Geometry: final body of the model. Coordinates: model frame, mm. A direction names the side the tool comes from. Give positions to 0.01 mm unless a question says otherwise; leave off trailing zeros. Loops run counter-clockwise (first coordinate to the right, second up) from the corner with the lowest first, then second, coordinate; pieces in that order, holes last.
from build123d import *

# Parameters (mm, degrees)
BOSS_EXTRUDE1_DEPTH = 6
SKETCH2_R           = 5.75
BOSS_EXTRUDE2_DEPTH = 12
SKETCH4_R           = 2
CUT_EXTRUDE2_DEPTH  = 21.199009877
SKETCH5_R           = 1.5
CUT_EXTRUDE3_DEPTH  = 6


with BuildPart() as part:
    # Sketch1 → Boss-Extrude1 (new body)
    with BuildSketch(Plane(origin=(0, 0, 0), x_dir=(0, 1, 0), z_dir=(0, 0, 1))):
        Polygon((0, 6.92820323), (-6, 3.464101615), (-6, -3.464101615), (0, -6.92820323), (6, -3.464101615), (6, 3.464101615), align=None)
    extrude(amount=BOSS_EXTRUDE1_DEPTH)

    # Sketch2 → Boss-Extrude2 (add)
    with BuildSketch(Plane(origin=(0, 0, 0), x_dir=(1, 0, 0), z_dir=(0, 0, -1))):
        with Locations(Location((0, 0, 0), (0, 0, 180))):
            Circle(SKETCH2_R)
    extrude(amount=BOSS_EXTRUDE2_DEPTH)

    # Sketch4 → Cut-Extrude2 (cut, through all)
    with BuildSketch(Plane(origin=(0, 0, -12), x_dir=(1, 0, 0), z_dir=(0, 0, -1))):
        with Locations(Location((0, 0, 0), (0, 0, 180))):
            Circle(SKETCH4_R)
    extrude(amount=-CUT_EXTRUDE2_DEPTH, mode=Mode.SUBTRACT)

    # Sketch5 → Cut-Extrude3 (cut)
    with BuildSketch(Plane(origin=(5.196152423, -3, 0), x_dir=(0.49999999999999506, 0.8660254037844415, 0), z_dir=(0.8660254037844415, -0.49999999999999506, 0))):
        with Locations((0, -6)):
            Circle(SKETCH5_R)
    extrude(amount=-CUT_EXTRUDE3_DEPTH, mode=Mode.SUBTRACT)


solid = part.part
Item 1: Draft query along X for faces 3 (the face through (6, -1, 0)), 4 (the face through (-1.908, 0.601, -3.126)), 5 (the face through (5.22, 2.96, 2.96)), 6 (the face through (3.807, -0.546, -5.549)). Return one class per face: +X half, -X half, draft (parallel to the pull), parting line (faces both ways), or undercut.
Values follow:
face 3: draft
face 4: undercut
face 5: +X half
face 6: undercut
Item 2: Pin query (flat end, axial travel): pin 1 (5 mm diameter, centred on x = 4.5, z = -7, fed in from -Y); pin 2 (5 mm diameter, centred on y = -2.5, z = -3, fed in from +X); pin 3 (5 mm diameter, centred on y = 4, z = 1.5, fed in from -X). Return the tip coordinate at first contact, or that it passes through.
Values follow:
pin 1: stops at y = -5.39
pin 2: stops at x = 5.75
pin 3: stops at x = -6.06
Item 3: Ray query, probe 1 along Y at (x, z) = (0, -1); probe 2 along Z at (x, y) = (3.25, -1.75); probe 3 along Y at (x, z) = (0, 1). Return the intervals inside material, ascending.
Values follow:
probe 1: y = -5.75 to -2, 2 to 5.75
probe 2: z = -12 to -7.5, -4.5 to 6
probe 3: y = -6 to -2, 2 to 6
Item 4: Section query D-D on x = -4. Return loops of the section in (y, z).
Values follow:
outline: (-5.07, 0) - (-4.13, 0) - (-4.13, -12) - (4.13, -12) - (4.13, 0) - (5.07, 0) - (5.07, 6) - (-5.07, 6) - close
Item 5: Section query C-C on y = 4.25. Return loops of the section in (x, z).
Values follow:
outline: (-4.47, 0) - (-3.87, 0) - (-3.87, -12) - (3.87, -12) - (3.87, 0) - (4.47, 0) - (4.47, 6) - (-4.47, 6) - close
Item 6: Section query B-B on z = 4. Return loops of the section in (x, y), plus the area to 3 significant figures.
Values follow:
outline: (-6.93, 0) - (-3.46, -6) - (3.46, -6) - (6.93, 0) - (3.46, 6) - (-3.46, 6) - close; hole circle Ø4 at (0, 0)
area: 112 mm2
Item 7: Section query A-A on x = 0. Return loops of the section in (y, z).
Values follow:
outline: (-6, 0) - (-5.75, 0) - (-5.75, -12) - (-2, -12) - (-2, 6) - (-6, 6) - close; (2, -12) - (5.75, -12) - (5.75, 0) - (6, 0) - (6, 6) - (2, 6) - close
Item 8: Set-up query: faces 1 (the face through (-3.09, 4.85, -5.92)), 2 (the face through (5.172, -3.042, 2.958)). Return all of +Z, -Z, +X, -X, +Y, -Y with unobstructed straight access to the full face (end or side cutting, diameter ignored); none if empty.
Values follow:
face 1: -Z
face 2: +Z, -Z, +X, -Y
